```python
from build123d import *

# Parameters (mm, degrees)
SALIENTE_EXTRUIR1_DEPTH = 10
REDONDEO1_R             = 10
REDONDEO2_R             = 2


with BuildPart() as part:
    # Croquis1 → Saliente-Extruir1 (new body)
    with BuildSketch(Plane(origin=(0, 0, 0), x_dir=(1, 0, 0), z_dir=(0, 1, 0))):
        with BuildLine():
            Line((-55.595903629, 23.860424538), (-55.595903629, -17.139575462))
            ThreePointArc((-55.595903629, -17.139575462), (-58.988591813, -15.192930957), (-61.826379426, -12.500957814))
            ThreePointArc((-61.826379426, -12.500957814), (-63.205175994, -12.346614438), (-63.411183057, -13.718643208))
            ThreePointArc((-63.411183057, -13.718643208), (-45.832647936, -24.756705017), (-25.595903629, -20.139575462))
            Line((-25.595903629, -20.139575462), (-25.595903629, 33.458404285))
            Line((-25.595903629, 33.458404285), (-57.189073116, 65.051573772))
            Line((-57.189073116, 65.051573772), (-91.850363788, 60.194112608))
            Line((-91.850363788, 60.194112608), (-86.576548855, 22.561854481))
            ThreePointArc((-86.576548855, 22.561854481), (-84.456782192, 20.844267935), (-82.595903629, 22.839423374))
            Line((-82.595903629, 22.839423374), (-82.595903629, 32.75382282))
            ThreePointArc((-82.595903629, 32.75382282), (-77.966029372, 39.682919314), (-69.79260277, 38.057123679))
            Line((-69.79260277, 38.057123679), (-55.595903629, 23.860424538))
        make_face()
    extrude(amount=SALIENTE_EXTRUIR1_DEPTH)

    # Redondeo1
    redondeo1_edges = [part.edges().sort_by_distance(p)[0] for p in [
        (-25.595903629, 5, -33.458404285),
        (-25.595903629, 5, 20.139575462),
        (-55.595903629, 5, -23.860424538),
        (-91.850363788, 5, -60.194112608),
        (-57.189073116, 5, -65.051573772),
    ]]
    fillet(redondeo1_edges, radius=REDONDEO1_R)

    # Redondeo2
    redondeo2_edges = [part.edges().sort_by_distance(p)[0] for p in [
        (-55.595903629, 5, 17.139575462),
    ]]
    fillet(redondeo2_edges, radius=REDONDEO2_R)


solid = part.part
```
Work out the finished part from the listing and answer in its coordinate system (mm). A direction names the side the tool comes from. Give positions to 0.01 mm unless a question says otherwise; leave off trailing zeros. Loops run counter-clockwise (first coordinate to the right, second up) from the corner with the lowest first, then second, coordinate; pieces in that order, holes last. Notation, with made-up numbers: M -22.5,-25.75 L 32.5,-25.75 A38 ccw 32.5,13.25 Z; hole C 30.5,-6 d7. An arc over 180 degrees is marked long. One line per item, written item: value. Start each with the question number.
1. Each of these flat-tipped pins is pushed along its axis until it touches: P1, Ø8, axis at x = -68.5, z = 9, coming from the -Y side; P2, Ø6, axis at x = -43.5, y = 7.5, coming from the -Z side; P3, Ø2, axis at x = -74, y = 7.5, coming from the +Z side (3 decimals); P4, Ø3, axis at y = 4, z = 1, coming from the -X side. Where does it stop, or does it pass through?
2. Find section A-A (y = 8). Give the vertices of the cut face in (x, z).
3. Determine the mould class of faces 1 (the face through (-40.92, 4.93, -48.78)), 2 (the face through (-88.547, 4.93, -36.62)), 3 (the face through (-60.36, 4.93, 14.05)) for opening direction X: released by +X, released by -X, zero draft, split by the parting line, or undercut.
4. Find the intervals of material crossed by probe 1 along X at (y, z) = (1.75, 6.5); probe 2 along Z at (x, y) = (-58.5, 4); probe 3 along X at (y, z) = (5.5, -21), in increasing order.
5. Which of the six approach directions +Z, -Z, +X, -X, +Y, -Y give full straight-line access (tool end or side, diameter ignored) to faces 4 (the face through (-56.66, 5.07, 15.5)), 5 (the face through (-82.596, 5, -28)), 6 (the face through (-51, 10, -20))?
6. Find section D-D (x = -36). Give the vertices of the cut face in (y, z), and give its area (3 significant figures).
7. Find section B-B (z = -39). Give the vertices of the cut face in (x, y), and give its area (3 significant figures).
8. Find section C-C (z = 7). Give the vertices of the cut face in (x, y).
Reported:
1. P1: passes through
1. P2: stops at z = -54.36
1. P3: stops at z = -39.955
1. P4: stops at x = -55.6
2. outline: M -90.46,-50.29 A10 ccw -81.95,-61.58 L -62.12,-64.36 A10 ccw -53.67,-61.53 L -28.52,-36.39 A10 ccw -25.6,-29.32 L -25.6,14.17 A10 ccw -32.27,23.6 A27.13 ccw -63.41,13.72 A1 ccw -61.83,12.5 A16.47 cw -58.76,15.36 A2 cw -55.6,13.73 L -55.6,-19.72 A10 cw -58.52,-26.79 L -69.79,-38.06 A7.5 cw -82.6,-32.75 L -82.6,-22.84 A2 ccw -86.58,-22.56 Z
3. face 1: released by +X
3. face 2: released by -X
3. face 3: undercut
4. probe 1: x = -55.6 to -25.6
4. probe 2: z = -64.2 to -26.76, 15.52 to 18.98
4. probe 3: x = -85.38 to -83.81, -55.68 to -25.6
5. face 4: +Y, -Y
5. face 5: +Z, +Y, -Y
5. face 6: +Z, -Z, +X, -X, +Y
6. outline: M 0,-43.86 L 10,-43.86 L 10,24.62 L 0,24.62 Z
6. area: 685 mm²
7. outline: M -88.88,0 L -79.25,0 L -79.25,10 L -88.88,10 Z; M -70.94,0 L -31.14,0 L -31.14,10 L -70.94,10 Z
7. area: 494 mm²
8. outline: M -55.6,0 L -25.6,0 L -25.6,10 L -55.6,10 Z
